```python
from build123d import *

# Parameters (mm, degrees)
BOSS_EXTRUDE1_DEPTH        = 22.5
M8_TAPPED_HOLE1_D          = 6.8
F_8_5_8_5_DIAMETER_HOLE2_D = 8.5


with BuildPart() as part:
    # Sketch1 → Boss-Extrude1 (new, symmetric)
    with BuildSketch(Plane(origin=(0, 0, 0), x_dir=(0, 0, -1), z_dir=(1, 0, 0))):
        Polygon((0, -40), (0, 0), (40, 0), (40, -4), (4, -4), (4, -40), align=None)
    extrude(amount=BOSS_EXTRUDE1_DEPTH, both=True)

    # M8 Tapped Hole1 (through all)
    with Locations(Plane(origin=(0, 0, 0), x_dir=(1, 0, 0), z_dir=(0, 1, 0))):
        with Locations((0, 22.5)):
            Hole(M8_TAPPED_HOLE1_D / 2)

    # Ø8.5 (8.5) Diameter Hole2 (through all)
    with Locations(Plane.XY):
        with Locations((-12.5, -22.5), (12.5, -22.5)):
            Hole(F_8_5_8_5_DIAMETER_HOLE2_D / 2)


solid = part.part
```
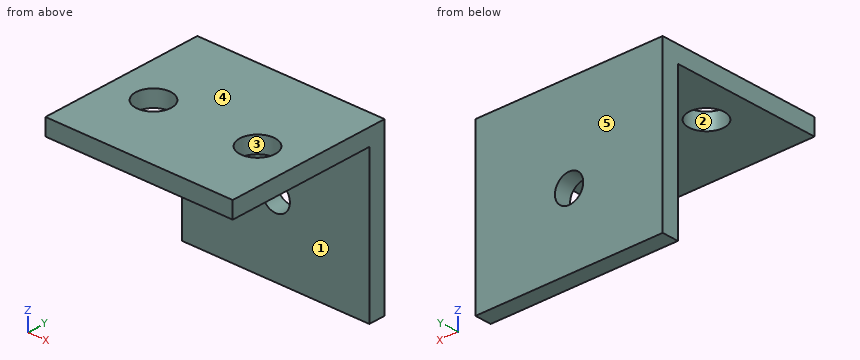
Could you check a few things on this model? Use its own coordinates, in mm. Face numbers are marked on the shaded views. A direction names the side the tool comes from. Coordinates: 2 decimals unless noted, no trailing zeros. Loops run counter-clockwise (first coordinate to the right, second up) from the corner with the lowest first, then second, coordinate; pieces in that order, holes last. Notation, with made-up numbers: M 81,57 L 96,57 A16 ccw 96,83 Z; hole C 67,50.5 d9. An arc over 180 degrees is marked long. Put each result on its own line as item: value. Start each with the question number.
(1) Suppose I cut it at C-C on y = -25. Please give me the cut outline in (x, z).
(2) Thinking about a two-plate mould opening in Y: for the marked faces 3, 4 and 5, which applies, pulls with the +Y half, pulls with the -Y half, needs draft (parallel to the pull), parting line crosses it, or undercut?
(3) For the marked faces 1 and 2, which set-ups out of +Z, -Z, +X, -X, +Y, -Y let a thin tool reach every point of the face, with its end or its side?
(4) Suppose I cut it at A-A on x = 12.5. Please give me the cut outline in (y, z).
(5) Suppose I cut it at D-D on x = 18. Please give me the cut outline in (y, z).
(6) Suppose I cut it at B-B on z = -22.5. Please give me the cut outline in (x, y).
(7) I need wall thicknesses on line 1 (Z direction, x = 0, y = -1); line 2 (X direction, y = -1.8, z = -22.5); line 3 (Y direction, x = 12.5, z = -2.9). Which ranges of each line are inside material? Lowest first, please. Write a range as from..to.
(8) Will these pins go through, and if not, where does the flat tip stop? P1, Ø11, axis at x = 2, y = -16, coming from the -Z side; P2, Ø5, axis at x = 12.5, y = -22.5, coming from the -Z side; P3, Ø6, axis at x = -5, z = -19.5, coming from the -Y side.
Solutions:
1. outline: M -22.5,-4 L -15.94,-4 L -15.94,0 L -22.5,0 Z; M -9.06,-4 L 9.06,-4 L 9.06,0 L -9.06,0 Z; M 15.94,-4 L 22.5,-4 L 22.5,0 L 15.94,0 Z
2. face 3: undercut
2. face 4: needs draft
2. face 5: pulls with the +Y half
3. face 1: -Z, +X, -X, -Y
3. face 2: +Z, -Z
4. outline: M -40,-4 L -26.75,-4 L -26.75,0 L -40,0 Z; M -18.25,-4 L -4,-4 L -4,-40 L 0,-40 L 0,0 L -18.25,0 Z
5. outline: M -40,-4 L -4,-4 L -4,-40 L 0,-40 L 0,0 L -40,0 Z
6. outline: M -22.5,-4 L -3.4,-4 L -3.4,0 L -22.5,0 Z; M 3.4,-4 L 22.5,-4 L 22.5,0 L 3.4,0 Z
7. line 1: z = -40..-25.9, -19.1..0
7. line 2: x = -22.5..-3.4, 3.4..22.5
7. line 3: y = -40..-26.75, -18.25..0
8. P1: stops at z = -4
8. P2: passes through
8. P3: stops at y = -4
